Geometry check sheet. Reference: the model listing, model coordinates, mm. Give positions to 0.01 mm unless a question says otherwise; leave off trailing zeros. Loops run counter-clockwise (first coordinate to the right, second up) from the corner with the lowest first, then second, coordinate; pieces in that order, holes last. Notation, with made-up numbers: (46, 36.25) -> (102, 36.25) arc R28 cw to (102, 65.25) -> close; hole circle Ø5 at (14.25, 59.25). An arc over 180 degrees is marked (long way). One line per question, with ' | ' between items.
Autodesk Fusion 360 part; units mm, degrees
sketch "スケッチ1" plane through (0, 0, 0) normal (0, 0, 1) x (1, 0, 0)
  line L0 (0, 0) -> (-12.5, 0)
  line L1 (-12.5, 0) -> (-12.5, 12)
  line L2 (-12.5, 12) -> (0, 12)
  line L3 (0, 12) -> (0, 0)
  line L4 (0, 0) -> (12.5, 0)
  line L5 (12.5, 0) -> (12.5, 12)
  line L6 (12.5, 12) -> (0, 12)
  line L7 (0, 12) -> (0, 0)
  line L8 (0, 0) -> (-12.5, 0)
  line L9 (-12.5, 0) -> (-12.5, -10.5)
  line L10 (-12.5, -10.5) -> (0, -10.5)
  line L11 (0, -10.5) -> (0, 0)
  line L12 (0, 0) -> (12.5, 0)
  line L13 (12.5, 0) -> (12.5, -10.5)
  line L14 (12.5, -10.5) -> (0, -10.5)
  line L15 (0, -10.5) -> (0, 0)
  line L16 (0, -10.5) -> (-9, -10.5)
  line L17 (-9, -10.5) -> (-9, -13)
  line L18 (-9, -13) -> (0, -13)
  line L19 (0, -13) -> (0, -10.5)
  line L20 (0, -10.5) -> (9, -10.5)
  line L21 (9, -10.5) -> (9, -13)
  line L22 (9, -13) -> (0, -13)
  line L23 (0, -13) -> (0, -10.5)
  line L24 (-12.5, 12) -> (-18.5, 12)
  line L25 (12.5, 12) -> (18.5, 12)
  arc A0 (-2.5, 28) -> (-18.5, 12) centre (-2.5, 12) ccw
  arc A1 (18.5, 12) -> (2.5, 28) centre (2.5, 12) ccw
  line L26 (-2.5, 28) -> (2.5, 28)
  circle A2 centre (-11, 7) radius 0.8
  circle A3 centre (-11, -7) radius 0.8
  circle A4 centre (11, -7) radius 0.8
  circle A5 centre (11, 7) radius 0.8
  circle A6 centre (0, 10.5) radius 6
  line L27 (0, 12) -> (0, 28)
  dimension "d1" = 6
  dimension "d2" = 12.5
  dimension "d3" = 12
  dimension "d4" = 28
  dimension "d5" = 1.6
  dimension "d6" = 7
  dimension "d7" = 3.5
  dimension "d8" = 3.5
  dimension "d9" = 2.5
  dimension "d10" = 12
  dimension "d11" = 10.5
  dimension "d17" = 22
extrude "押し出し1" add sketch "スケッチ1" along normal blind 0.6 contours L0 L8 L9 L10 L11 L15 L16 | L0 L1 L2 L3 L7 L8 A6 | L3 L4 L5 L6 L7 L12 A6 | L4 L11 L12 L13 L14 L15 L20 | L10 L16 L17 L18 L19 L23 | L14 L19 L20 L21 L22 L23 | L2 L24 A0 L26 A6 L27 | L6 L25 A1 L26 A6 L27
fillet "フィレット1" radius 3 2 edges at (-18.5, 12, 0.3) (18.5, 12, 0.3)
fillet "フィレット1" radius 2 2 edges at (-12.5, 12, 0.3) (12.5, 12, 0.3)
fillet "フィレット1" radius 1 6 edges at (-12.5, -10.5, 0.3) (-9, -10.5, 0.3) (-9, -13, 0.3) (9, -13, 0.3) (9, -10.5, 0.3) (12.5, -10.5, 0.3)
Item 1: Sectioned sample at B-B (z = 0.1). Record the cut outline in (x, y).
Result:
outline: (-18.07, 15.69) arc R3 ccw to (-15.15, 12) -> (-14.5, 12) arc R2 cw to (-12.5, 10) -> (-12.5, -9.5) arc R1 ccw to (-11.5, -10.5) -> (-10, -10.5) arc R1 cw to (-9, -11.5) -> (-9, -12) arc R1 ccw to (-8, -13) -> (8, -13) arc R1 ccw to (9, -12) -> (9, -11.5) arc R1 cw to (10, -10.5) -> (11.5, -10.5) arc R1 ccw to (12.5, -9.5) -> (12.5, 10) arc R2 cw to (14.5, 12) -> (15.15, 12) arc R3 ccw to (18.07, 15.69) arc R16 ccw to (2.5, 28) -> (-2.5, 28) arc R16 ccw to start; hole circle Ø1.6 at (-11, -7); hole circle Ø1.6 at (-11, 7); hole circle Ø12 at (0, 10.5); hole circle Ø1.6 at (11, -7); hole circle Ø1.6 at (11, 7)
Item 2: Sectioned sample at A-A (y = -7). Record the cut outline in (x, z), plus the area to 3 significant figures.
Result:
outline: (-12.5, 0) -> (-11.8, 0) -> (-11.8, 0.6) -> (-12.5, 0.6) -> close; (-10.2, 0) -> (10.2, 0) -> (10.2, 0.6) -> (-10.2, 0.6) -> close; (11.8, 0) -> (12.5, 0) -> (12.5, 0.6) -> (11.8, 0.6) -> close | area: 13.1 mm2
Item 3: Sectioned sample at C-C (y = 7). Record the cut outline in (x, z), plus the area to 3 significant figures.
Result:
outline: (-12.5, 0) -> (-11.8, 0) -> (-11.8, 0.6) -> (-12.5, 0.6) -> close; (-10.2, 0) -> (-4.87, 0) -> (-4.87, 0.6) -> (-10.2, 0.6) -> close; (4.87, 0) -> (10.2, 0) -> (10.2, 0.6) -> (4.87, 0.6) -> close; (11.8, 0) -> (12.5, 0) -> (12.5, 0.6) -> (11.8, 0.6) -> close | area: 7.23 mm2
Item 4: Sectioned sample at D-D (x = 11). Record the cut outline in (y, z).
Result:
outline: (-10.5, 0) -> (-7.8, 0) -> (-7.8, 0.6) -> (-10.5, 0.6) -> close; (-6.2, 0) -> (6.2, 0) -> (6.2, 0.6) -> (-6.2, 0.6) -> close; (7.8, 0) -> (25.56, 0) -> (25.56, 0.6) -> (7.8, 0.6) -> close
Item 5: Scan lines: probe 1 along Y at (x, z) = (11, 0.2); probe 2 along X at (y, z) = (-3, 0.1); probe 3 along X at (y, z) = (-7.5, 0.2). Record each from-to range of solid material in increasing order.
Result:
probe 1: -10.5 to -7.8, -6.2 to 6.2, 7.8 to 25.56 | probe 2: -12.5 to 12.5 | probe 3: -12.5 to -11.62, -10.38 to 10.38, 11.62 to 12.5
Item 6: Depth check by flat-ended pin: pin 1 Ø1.8 at (x, y) = (11, 7) entering from +Z. Enter the tip coordinate at first touch or a pass-through.
Result:
pin 1: z = 0.6
